```python
from build123d import *

# Parameters (mm, degrees)
F0_R     = 247.5
F0_R_2   = 7.5
F1_DEPTH = 6


with BuildPart() as f1:
    # F0 (on Front) → F1 (new body)
    with BuildSketch(Plane.XZ):
        Circle(F0_R)
        with BuildLine():
            ThreePointArc((-54.014982, -207.906888), (-87.753912, -171.700505), (-100, -123.75))
            Line((-100, -123.75), (-30, -123.75))
            ThreePointArc((-30, -123.75), (-27.079055, -136.662194), (-18.885016, -147.060002))
            Line((-18.885016, -147.060002), (-54.014982, -207.906888))
        make_face(mode=Mode.SUBTRACT)
        with BuildLine():
            Line((30, -123.75), (100, -123.75))
            ThreePointArc((100, -123.75), (86.588738, -173.773898), (49.952192, -210.380125))
            Line((49.952192, -210.380125), (14.952174, -149.758316))
            ThreePointArc((14.952174, -149.758316), (25.966952, -138.773894), (30, -123.75))
        make_face(mode=Mode.SUBTRACT)
        with Locations((0, -123.75)):
            Circle(F0_R_2, mode=Mode.SUBTRACT)
        with BuildLine():
            Line((-18.960726, -100.50154), (-54.096123, -39.645247))
            ThreePointArc((-54.096123, -39.645247), (1.641257, -23.76347), (56.827358, -41.466032))
            Line((56.827358, -41.466032), (21.437345, -102.763332))
            ThreePointArc((21.437345, -102.763332), (1.677002, -93.796909), (-18.960726, -100.50154))
        make_face(mode=Mode.SUBTRACT)
    extrude(amount=F1_DEPTH)


solid = f1.part
```
The model under review builds one solid part; all positions refer to its coordinate system, in mm. A direction names the side the tool comes from. Give positions to 0.01 mm unless a question says otherwise; leave off trailing zeros. Write each loop counter-clockwise with the first axis right and the second up, starting at its lowest first coordinate (ties: lowest second). Pieces come first, ordered by that corner, then holes.
(1) The part is to be moulded in two halves that separate along X. For faces 1 (the flat face through (-36.204, -2.958, -177.058)), 2 (the cylindrical face through (-32.22, -2.958, 245.394)), 3 (the flat face through (-3, 0, 3)), say which applies: released by +X, released by -X, zero draft, split by the parting line, or undercut.
(2) Tool access review of faces 4 (the flat face through (-3, -6, 3)), 5 (the cylindrical face through (25.86, -2.96, -138.96)): name each direction out of +Z, -Z, +X, -X, +Y, -Y from which nothing blocks a thin tool from reaching the whole face with its end or side.
(3) Consider section D-D, the plane z = -193.5. Give the boundary of the cut face in (x, y), and give its area (3 significant figures).
(4) Consider section A-A, the plane y = -2.4. Give the boundary of the cut face in (x, z).
(5) To check wall thickness, follow L1, parallel to Z at x = 0, y = -1.45; L2, parallel to Z at x = -50.5, y = -3.15; L3, parallel to X at y = -3.05, z = -186. State the ranges of each line that lie inside material, in increasing order.
(6) Consider section B-B, the plane x = 0. Give the boundary of the cut face in (y, z).
(7) Consider section C-C, the plane x = -66.5. Give the boundary of the cut face in (y, z), and give its area (3 significant figures).
(8) For P1, Ø1, axis at x = 167.5, y = -2.5, coming from the -Z side; P2, Ø1.5, axis at y = -5, z = 125.5, coming from the -X side, all flat-tipped, find the tip position at first contact; note any pin that passes through.
Returned:
1. face 1: undercut
1. face 2: split by the parting line
1. face 3: zero draft
2. face 4: +Z, -Z, +X, -X, -Y
2. face 5: +Y, -Y
3. outline: (-154.32, -6) - (-71.66, -6) - (-71.66, 0) - (-154.32, 0) - close; (-45.7, -6) - (40.21, -6) - (40.21, 0) - (-45.7, 0) - close; (71.66, -6) - (154.32, -6) - (154.32, 0) - (71.66, 0) - close
3. area: 1,510 mm2
4. outline: circle Ø495 at (0, 0); hole (-100, -123.75) arc R100 ccw to (-54.01, -207.91) - (-18.89, -147.06) arc R30 cw to (-30, -123.75) - close; hole (-54.1, -39.65) - (-18.96, -100.5) arc R30 cw to (21.44, -102.76) - (56.83, -41.47) arc R100 ccw to start; hole circle Ø15 at (0, -123.75); hole (14.95, -149.76) - (49.95, -210.38) arc R100 ccw to (100, -123.75) - (30, -123.75) arc R30 cw to start
5. L1: z = -247.5 to -131.25, -116.25 to -93.75, -23.75 to 247.5
5. L2: z = -242.29 to -201.82, -123.75 to -45.87, -37.44 to 242.29
5. L3: x = -163.28 to -78.26, -41.37 to 35.88, 78.26 to 163.28
6. outline: (-6, -247.5) - (0, -247.5) - (0, -131.25) - (-6, -131.25) - close; (-6, -116.25) - (0, -116.25) - (0, -93.75) - (-6, -93.75) - close; (-6, -23.75) - (0, -23.75) - (0, 247.5) - (-6, 247.5) - close
7. outline: (-6, -238.4) - (0, -238.4) - (0, -198.43) - (-6, -198.43) - close; (-6, -123.75) - (0, -123.75) - (0, 238.4) - (-6, 238.4) - close
7. area: 2,410 mm2
8. P1: stops at z = -182.67
8. P2: stops at x = -213.76
